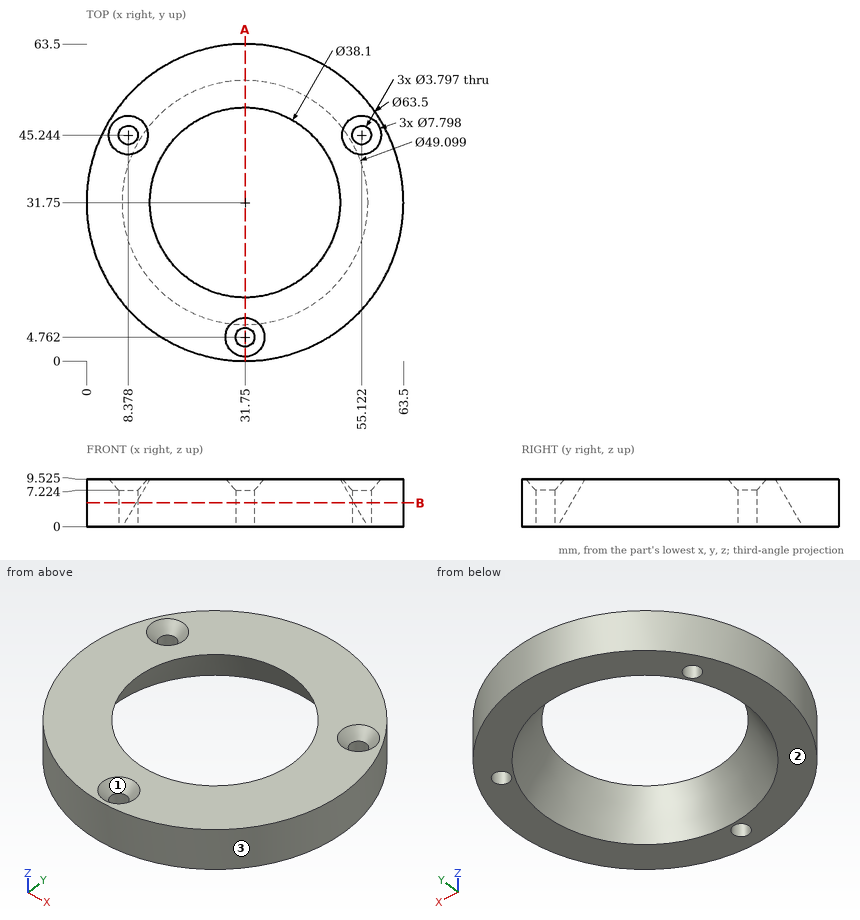
Design review of the part shown in the three views and the two pictorial views. Dimensions are in mm from the part's minimum x, y and z. Coordinates: 2 decimals unless noted, no trailing zeros. Write each loop counter-clockwise with the first axis right and the second up, starting at its lowest first coordinate (ties: lowest second). Pieces come first, ordered by that corner, then holes. Notation, with made-up numbers: (16, -39.75) -> (43, -39.75) arc R25 cw to (43, -16.75) -> close; hole circle Ø10 at (25, 37.5). An arc over 180 degrees is marked (long way). Answer in a Markdown table with one row per item.
1. We need section A-A, the plane x = 31.75. State the section outline as (y, z) points (1 decimal), and give its area (3 significant figures).
Answers below:
| item | result |
|---|---|
| outline | (0, 0) -> (2.9, 0) -> (2.9, 7.2) -> (0.9, 9.5) -> (0, 9.5) -> close; (6.7, 0) -> (7.2, 0) -> (12.7, 9.5) -> (8.7, 9.5) -> (6.7, 7.2) -> close; (50.8, 9.5) -> (56.3, 0) -> (63.5, 0) -> (63.5, 9.5) -> close |
| area | 149 mm^2 |
2. Wall thickness on probe 1 along Y at (x, z) = (31.75, 4.5) (1 decimal); probe 2 along X at (y, z) = (48, 8.5) (1 decimal); probe 3 along Y at (x, z) = (33, 6.5) (1 decimal): over which ranges is each line inside the solid? List them lowest first. Write a range as [from, to].
Answers below:
| item | result |
|---|---|
| probe 1 | y = [0, 2.9], [6.7, 9.8], [53.7, 63.5] |
| probe 2 | x = [4.5, 7.2], [9.6, 20.7], [42.8, 53.9], [56.3, 59] |
| probe 3 | y = [0, 3.3], [6.2, 11], [52.5, 63.5] |
3. Clearance check with flat-ended pins moving along their axes: pin 1 Ø1.5 at (x, y) = (9, 45) entering from +Z; pin 2 Ø5 at (x, z) = (48, 6.5) entering from -Y; pin 3 Ø1.5 at (y, z) = (28, 6.5) entering from +X; pin 4 Ø3 at (x, z) = (41.5, 5) entering from -Y. State where each tip first meets the part, or that it passes through.
Answers below:
| item | result |
|---|---|
| pin 1 | passes through |
| pin 2 | stops at y = 3.13 |
| pin 3 | stops at x = 63.36 |
| pin 4 | stops at y = 1.09 |
4. Draft analysis for pull direction X (two halves, no side actions). For the marked faces 1, 2 and 3, state which applies: +X half, -X half, draft (parallel to the pull), parting line (faces both ways), or undercut.
Answers below:
| item | result |
|---|---|
| face 1 | undercut |
| face 2 | draft |
| face 3 | parting line |
5. We need section B-B, the plane z = 4.75. State the section outline as (x, y) points.
Answers below:
| item | result |
|---|---|
| outline | circle Ø63.5 at (31.75, 31.75); hole circle Ø3.8 at (8.38, 45.24); hole circle Ø43.61 at (31.75, 31.75); hole circle Ø3.8 at (31.75, 4.76); hole circle Ø3.8 at (55.12, 45.24) |
